For this review, take the finished solid that the model builds, in its own axes (mm). Face numbers are marked on the shaded views. A direction names the side the tool comes from. Give positions to 0.01 mm unless a question says otherwise; leave off trailing zeros. Loops run counter-clockwise (first coordinate to the right, second up) from the corner with the lowest first, then second, coordinate; pieces in that order, holes last. Notation, with made-up numbers: (29, 13) -> (63, 13) arc R14 cw to (63, 37) -> close; hole circle Ø2 at (64, 70). An arc over 180 degrees is marked (long way). Answer as CSV lines item,"result". Start each with the question number.
Item 1: Machinability: for the marked faces 1 and 2, which of the approach directions +Z, -Z, +X, -X, +Y, -Y give a long, thin tool a straight path to every point of the face, cutting with its end or side? Answer none if there is none.
Item 2: Add section A-A on z = -16. State the section outline as (x, y) points.
Item 3: Add section B-B on x = 15.5. State the section outline as (y, z) points, plus the area to 3 significant figures.
Item 4: Clearance check with flat-ended pins moving along their axes: P1, Ø1.5, axis at x = -18, y = 1, coming from the +Z side; P2, Ø0.9, axis at y = 1.5, z = 28, coming from the +X side; P3, Ø11, axis at x = 0.5, z = -9, coming from the +Y side; P4, Ø1.9, axis at x = -15.77, z = 15.2, coming from the -Y side. State where each tip first meets the part, or that it passes through.
Item 5: The part is to be moulded in two halves that separate along X. For the marked faces 3 and 4, say which applies: +X half, -X half, draft (parallel to the pull), parting line (faces both ways), or undercut.
Item 6: Add section D-D on y = 1.55. State the section outline as (x, z) points, plus the area to 3 significant figures.
Item 7: For L1, parallel to Z at x = -16.5, y = 0.45; L2, parallel to X at y = 1.15, z = 16; L3, parallel to X at y = 1.6, z = -14, list the stretches that pass through material, from the lowest coordinate up. Write a range as from..to.
Item 8: Add section C-C on x = 5. State the section outline as (y, z) points, plus the area to 3 significant figures.
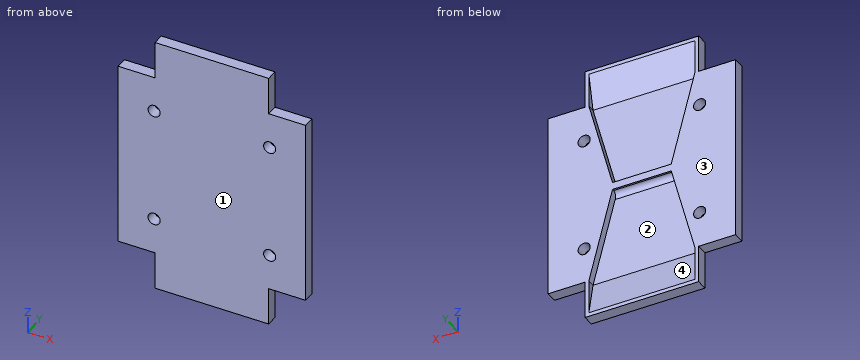
Autodesk Inventor part; units mm, degrees
ref_plane "YZ Plane" through (0, 0, 0) normal (1, 0, 0) x (0, 1, 0)
ref_plane "XZ Plane" through (0, 0, 0) normal (0, 1, 0) x (-1, 0, 0)
ref_plane "XY Plane" through (0, 0, 0) normal (0, 0, 1) x (1, 0, 0)
sketch "Sketch1" plane through (0, 0, 0) normal (0, 1, 0) x (-1, 0, 0)
  line L0 (25.2706, 24.6953) -> (-24.2294, 24.6953)
  line L1 (-24.2294, 24.6953) -> (-24.2294, -24.8047)
  line L2 (-24.2294, -24.8047) -> (25.2706, -24.8047)
  line L3 (25.2706, -24.8047) -> (25.2706, 24.6953)
  circle A0 centre (15.7706, 15.1953) radius 1.6
  circle A1 centre (15.7706, -15.3047) radius 1.6
  circle A2 centre (-14.7294, 15.1953) radius 1.6
  circle A3 centre (-14.7294, -15.3047) radius 1.6
  dimension "d17" = 49.5
  dimension "d18" = 49.5
  dimension "d19" = 3.2
  dimension "d20" = 3.2
  dimension "d21" = 30.5
  dimension "d22" = 9.5
  dimension "d23" = 9.5
  dimension "d24" = 9.5
  dimension "d25" = 9.5
  dimension "d26" = 3.2
  dimension "d27" = 3.2
  dimension "d28" = 30.5
  dimension "d29" = 30.5
  dimension "d30" = 30.5
  dimension "d31" = 9.5
  dimension "d32" = 9.5
  dimension "d33" = 9.5
  dimension "d34" = 9.5
extrude "Extrusion1" add sketch "Sketch1" along normal blind 3
sketch "Sketch2" plane through (0, 3, 0) normal (0, 1, 0) x (1, 0, 0)
  line L0 (-25.2706, -24.6953) -> (24.2294, -24.6953)
  line L1 (-0.5206, -24.6953) -> (-0.5206, 24.8047)
  line L2 (24.2294, 24.8047) -> (-25.2706, 24.8047)
  line L3 (-0.5206, -24.6953) -> (-15.5206, -24.6953)
  line L4 (-15.5206, -24.6953) -> (-15.5206, -34.6953)
  line L5 (-15.5206, -34.6953) -> (14.4794, -34.6953)
  line L6 (14.4794, -34.6953) -> (14.4794, -24.6953)
  line L7 (14.4794, -24.6953) -> (-0.5206, -24.6953)
  line L8 (-0.5206, 24.8047) -> (-15.5206, 24.8047)
  line L9 (-15.5206, 24.8047) -> (-15.5206, 34.8047)
  line L10 (-15.5206, 34.8047) -> (14.4794, 34.8047)
  line L11 (14.4794, 34.8047) -> (14.4794, 24.8047)
  line L12 (-0.5206, 24.8047) -> (14.4794, 24.8047)
  point P0 (0, 0)
  dimension "d37" = 15
  dimension "d38" = 10
  dimension "d39" = 30
  dimension "d40" = 15
  dimension "d41" = 10
  dimension "d42" = 30
extrude "Extrusion2" add sketch "Sketch2" against normal blind 3
sketch "Sketch3" plane through (0, 3, 0) normal (0, 1, 0) x (1, 0, 0)
  line L0 (-15.5206, -34.6953) -> (14.4794, -34.6953)
  line L1 (-0.5206, -34.6953) -> (-0.5206, 34.8047)
  line L2 (-15.5206, 34.8047) -> (14.4794, 34.8047)
  line L3 (-0.5206, -34.6953) -> (-0.5206, -33.6953)
  line L4 (-0.5206, -33.6953) -> (-14.5206, -33.6953)
  line L5 (-14.5206, -33.6953) -> (-14.5206, -24.6953)
  line L6 (-0.5206, -33.6953) -> (13.4794, -33.6953)
  line L7 (13.4794, -33.6953) -> (13.4794, -24.6953)
  line L8 (-0.5206, 34.8047) -> (-0.5206, 33.8047)
  line L9 (-0.5206, 33.8047) -> (-14.5206, 33.8047)
  line L10 (-14.5206, 33.8047) -> (-14.5206, 24.8047)
  line L11 (-0.5206, 33.8047) -> (13.4794, 33.8047)
  line L12 (13.4794, 33.8047) -> (13.4794, 24.8047)
  circle A0 centre (-0.5206, 0.0547) radius 7.5
  line L13 (-14.5206, -24.6953) -> (-8.0206, 0.0547)
  line L14 (-14.5206, 24.8047) -> (-8.0206, 0.0547)
  line L15 (13.4794, -24.6953) -> (6.9794, 0.0547)
  line L16 (13.4794, 24.8047) -> (6.9794, 0.0547)
  point P0 (0, 0)
  dimension "d45" = 1
  dimension "d46" = 14
  dimension "d47" = 14
  dimension "d48" = 1
  dimension "d49" = 14
  dimension "d50" = 14
  dimension "d51" = 15
extrude "Extrusion3" cut sketch "Sketch3" against normal blind 2
sketch "Sketch4" plane through (0, 1, 0) normal (0, 1, 0) x (1, 0, 0)
  point P0 (0, 0)
sketch "Sketch5" plane through (0, 1, 0) normal (0, 1, 0) x (1, 0, 0)
  line L0 (-14.5206, -24.6953) -> (-8.0206, 0.0547)
  line L1 (6.9794, 0.0547) -> (13.4794, -24.6953)
  line L2 (-8.0206, 0.0547) -> (6.9794, 0.0547)
  line L3 (-8.0206, 0.0547) -> (-8.2747, 1.0219)
  line L4 (-8.0206, 0.0547) -> (-14.5206, 24.8047)
  line L5 (-8.0206, 0.0547) -> (-8.2747, -0.9125)
  line L6 (13.4794, 24.8047) -> (6.9794, 0.0547)
  line L7 (6.9794, 0.0547) -> (7.2334, 1.0219)
  line L8 (6.9794, 0.0547) -> (7.2334, -0.9125)
  line L9 (7.2334, -0.9125) -> (-8.2747, -0.9125)
  line L10 (-8.2747, 1.0219) -> (7.2334, 1.0219)
  point P0 (0, 0)
  dimension "d56" = 1
  dimension "d57" = 1
  dimension "d58" = 1
  dimension "d59" = 1
extrude "Extrusion4" add sketch "Sketch5" along normal blind 2
fillet "Face Fillet3" radius 1.5 1 edges at (-0.5206, 1, -1.0219)
fillet "Face Fillet4" radius 1.5 1 edges at (-0.5206, 1, 0.9125)
sketch "Sketch6" plane through (-14.5206, 3, -24.8047) normal (1, 0, 0) x (0, 0, -1)
  line L0 (-22.2828, -2) -> (0, -2)
  line L1 (9, 0) -> (9, -2)
  line L2 (0, -2) -> (9, -2)
  line L3 (9, -2) -> (9, 0)
  line L4 (9, 0) -> (0, -2)
  line L5 (-58.5, 0) -> (-49.5, 0)
  line L6 (-58.5, 0) -> (-58.5, -2)
  line L7 (-58.5, -2) -> (-49.5, -2)
  line L8 (-49.5, -2) -> (-58.5, 0)
  point P0 (-24.8047, -3)
extrude "Extrusion5" add sketch "Sketch6" along normal blind 28.9875
properties material "PC/ABS Plastic"
Computed values:
1,face 1,"+Z, -Z, +X, -X, -Y"
1,face 2,"+Y"
2,outline,"(-25.27, 0) -> (-17.21, 0) -> (-17.21, 3) -> (-25.27, 3) -> close; (-14.33, 0) -> (13.29, 0) -> (13.29, 3) -> (11.17, 3) -> (11.17, 1) -> (-12.21, 1) -> (-12.21, 3) -> (-14.33, 3) -> close; (16.17, 0) -> (24.23, 0) -> (24.23, 3) -> (16.17, 3) -> close"
3,outline,"(0, -24.8) -> (3, -24.8) -> (3, -16.71) -> (0, -16.71) -> close; (0, -13.9) -> (3, -13.9) -> (3, 13.79) -> (0, 13.79) -> close; (0, 16.6) -> (3, 16.6) -> (3, 24.7) -> (0, 24.7) -> close"
3,area,"132 mm²"
4,P1,"z = 24.7"
4,P2,"x = 14.48"
4,P3,"y = 1"
4,P4,"through"
5,face 3,"draft"
5,face 4,"undercut"
6,outline,"(-25.27, -24.8) -> (-15.52, -24.8) -> (-15.52, -34.8) -> (14.48, -34.8) -> (14.48, -24.8) -> (24.23, -24.8) -> (24.23, 24.7) -> (14.48, 24.7) -> (14.48, 34.7) -> (-15.52, 34.7) -> (-15.52, 24.7) -> (-25.27, 24.7) -> close; hole circle Ø3.2 at (-15.77, -15.3); hole circle Ø3.2 at (-15.77, 15.2); hole (-14.52, -27.28) -> (13.48, -27.28) -> (13.48, -24.8) -> (7.32, -1.36) -> (-8.36, -1.36) -> (-14.52, -24.8) -> close; hole (-14.52, 24.7) -> (-8.36, 1.25) -> (7.32, 1.25) -> (13.48, 24.7) -> (13.48, 27.17) -> (-14.52, 27.17) -> close; hole circle Ø3.2 at (14.73, -15.3); hole circle Ø3.2 at (14.73, 15.2)"
6,area,"1,860 mm²"
7,L1,"-24.8..-16.73, -13.88..13.77, 16.62..24.7"
7,L2,"-25.27..-17.15, -14.39..-12.24, 11.2..13.35, 16.11..24.23"
7,L3,"-25.27..-16.7, -14.84..-11.68, 10.64..13.8, 15.66..24.23"
8,outline,"(0, -34.8) -> (3, -34.8) -> (3, -33.8) -> (1, -24.8) -> (1, -2.52) arc R1.5 cw to (2.5, -1.02) -> (3, -1.02) -> (3, 0.91) -> (2.5, 0.91) arc R1.5 cw to (1, 2.41) -> (1, 24.7) -> (3, 33.7) -> (3, 34.7) -> (0, 34.7) -> close"
8,area,"96.3 mm²"
